```python
from build123d import *

# Parameters (mm, degrees)
SKETCH_1_R      = 2
SKETCH_1_R_2    = 1
EXTRUDE_1_DEPTH = 2
FILLET_1_R      = 2


with BuildPart() as part:
    # 草图1 → 凸台-拉伸1 (new body)
    with BuildSketch(Plane.XY):
        with BuildLine():
            Line((-22.340449028, 112.565520938), (-22.340449028, 35.565520938))
            Line((-22.340449028, 35.565520938), (-41.340449028, 35.565520938))
            Line((-41.340449028, 35.565520938), (-41.340449028, 19.565520938))
            Line((-41.340449028, 19.565520938), (14.659550972, 19.565520938))
            Line((14.659550972, 19.565520938), (14.659550972, 35.565520938))
            Line((14.659550972, 35.565520938), (-4.340449028, 35.565520938))
            Line((-4.340449028, 35.565520938), (-4.340449028, 112.565520938))
            ThreePointArc((-4.340449028, 112.565520938), (-13.340449028, 121.565520938), (-22.340449028, 112.565520938))
        make_face()
        with Locations((-33.340449028, 27.565520938)):
            Circle(SKETCH_1_R, mode=Mode.SUBTRACT)
        with Locations(Location((6.659550972, 27.565520938, 0), (0, 0, 180))):
            Circle(SKETCH_1_R, mode=Mode.SUBTRACT)
        with Locations((-7.340449028, 112.565520938)):
            Circle(SKETCH_1_R_2, mode=Mode.SUBTRACT)
        with Locations(Location((-19.340449028, 112.565520938, 0), (0, 0, 180))):
            Circle(SKETCH_1_R_2, mode=Mode.SUBTRACT)
        with Locations((-13.340449028, 47.565520938)):
            Circle(SKETCH_1_R, mode=Mode.SUBTRACT)
    extrude(amount=EXTRUDE_1_DEPTH)

    # 圆角1
    fillet_1_edges = [part.edges().sort_by_distance(p)[0] for p in [
        (-41.340449028, 19.565520938, 1),
        (-41.340449028, 35.565520938, 1),
        (-22.340449028, 35.565520938, 1),
        (-4.340449028, 35.565520938, 1),
        (14.659550972, 35.565520938, 1),
        (14.659550972, 19.565520938, 1),
    ]]
    fillet(fillet_1_edges, radius=FILLET_1_R)


solid = part.part
```
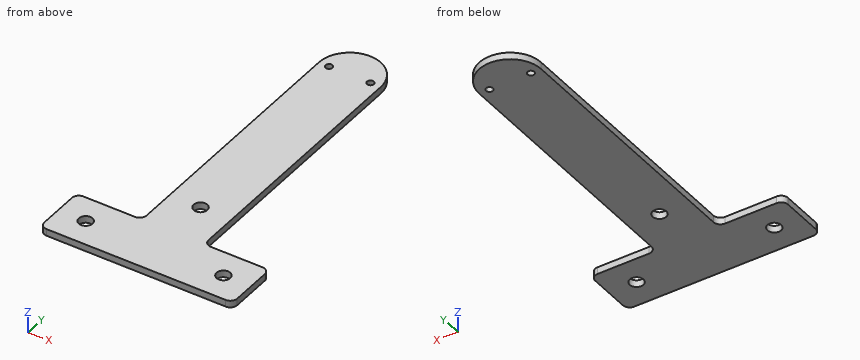
Build history of the part. All positions in model axes, mm. Give positions to 0.01 mm unless a question says otherwise; leave off trailing zeros. Loops run counter-clockwise (first coordinate to the right, second up) from the corner with the lowest first, then second, coordinate; pieces in that order, holes last. Notation, with made-up numbers: (-22, 81.25) - (4, 81.25) arc R11 cw to (4, 97.25) - close; hole circle Ø11 at (-14.75, -13). An arc over 180 degrees is marked (long way). Use a Markdown table: item, result.
(1) Drop flat-ended pins along their axis: pin 1 Ø1 at (y, z) = (102, 1.5) entering from -X; pin 2 Ø0.6 at (y, z) = (91.5, 1) entering from +X; pin 3 Ø1 at (x, z) = (-5, 0.5) entering from +Y; pin 4 Ø6.5 at (x, y) = (-13.34, 47.57) entering from -Z. Give the stop position or say it passes through.
Taken from the geometry:
| item | result |
|---|---|
| pin 1 | x = -22.34 |
| pin 2 | x = -4.34 |
| pin 3 | y = 116.98 |
| pin 4 | z = 0 |
(2) Wall check: line 1 along Y through (x, z) = (6.5, 1.65); line 2 along X through (y, z) = (26, 1.35); line 3 along X through (y, z) = (91, 0.8). Give the ranges that are in metal, low to high.
Taken from the geometry:
| item | result |
|---|---|
| line 1 | 19.57 to 25.57, 29.56 to 35.57 |
| line 2 | -41.34 to -34.59, -32.1 to 5.41, 7.9 to 14.66 |
| line 3 | -22.34 to -4.34 |
(3) Band-saw the part on D-D (x = -38). Give the cut face in (y, z).
Taken from the geometry:
| item | result |
|---|---|
| outline | (19.57, 0) - (35.57, 0) - (35.57, 2) - (19.57, 2) - close |
(4) Band-saw the part on A-A (x = 7). Give the cut face in (y, z), and give its area (3 significant figures).
Taken from the geometry:
| item | result |
|---|---|
| outline | (19.57, 0) - (25.59, 0) - (25.59, 2) - (19.57, 2) - close; (29.54, 0) - (35.57, 0) - (35.57, 2) - (29.54, 2) - close |
| area | 24.1 mm2 |
(5) Band-saw the part on B-B (z = 0.6). Give the cut face in (x, y).
Taken from the geometry:
| item | result |
|---|---|
| outline | (-41.34, 21.57) arc R2 ccw to (-39.34, 19.57) - (12.66, 19.57) arc R2 ccw to (14.66, 21.57) - (14.66, 33.57) arc R2 ccw to (12.66, 35.57) - (-2.34, 35.57) arc R2 cw to (-4.34, 37.57) - (-4.34, 112.57) arc R9 ccw to (-22.34, 112.57) - (-22.34, 37.57) arc R2 cw to (-24.34, 35.57) - (-39.34, 35.57) arc R2 ccw to (-41.34, 33.57) - close; hole circle Ø4 at (-33.34, 27.57); hole circle Ø2 at (-19.34, 112.57); hole circle Ø4 at (-13.34, 47.57); hole circle Ø2 at (-7.34, 112.57); hole circle Ø4 at (6.66, 27.57) |
(6) Band-saw the part on C-C (y = 104.5). Give the cut face in (x, z), and give its area (3 significant figures).
Taken from the geometry:
| item | result |
|---|---|
| outline | (-22.34, 0) - (-4.34, 0) - (-4.34, 2) - (-22.34, 2) - close |
| area | 36.0 mm2 |
